```python
from build123d import *

# Parameters (mm, degrees)
F1_DEPTH       = 17
F3_W           = 0.5
F3_H           = 0.6
F4_DEPTH       = 5
F3_W_2         = 1
F3_H_2         = 1.2
F5_DEPTH       = 7
F7_W           = 2.5
F7_H           = 0.8
F8_DEPTH       = 37.3
F6_W           = 37.3
F6_H           = 12.9
F9_DEPTH       = 0.8
F10_W          = 9.4
F10_H          = 0.8
F11_DEPTH      = 36.4
F12_DEPTH      = 25
F12_DEPTH_BACK = 36.401
F13_DEPTH      = 0.901
F14_R          = 2


with BuildPart() as f1:
    # F0 (on Top) → F1 (new body)
    with BuildSketch(Plane.XY):
        Polygon((-0.9, 0), (0, 0), (0, 14), (35.5, 14), (35.5, 0), (36.4, 0), (36.4, 14.9), (-0.9, 14.9), align=None)
    extrude(amount=F1_DEPTH)

    # F3 (on offset) → F4 (join)
    with BuildSketch(Plane.XZ.offset(-1)):
        with Locations((0.25, 14.7)):
            Rectangle(F3_W, F3_H)
        with Locations((0.25, 7.05)):
            Rectangle(F3_W, F3_H)
    extrude(amount=-F4_DEPTH)

    # F3 (on offset) → F5 (cut)
    with BuildSketch(Plane.XZ.offset(-1)):
        with Locations((36, 14.8)):
            Rectangle(F3_W_2, F3_H_2)
        with Locations((36, 6.8)):
            Rectangle(F3_W_2, F3_H_2)
    extrude(amount=-F5_DEPTH, mode=Mode.SUBTRACT)

    # F7 (on face) → F8 (join, through all)
    with BuildSketch(Plane.YZ.offset(36.4)):
        with Locations((13.65, 4.6)):
            Rectangle(F7_W, F7_H)
    extrude(amount=-F8_DEPTH)

    # F6 (on face) → F9 (join)
    with BuildSketch(Plane.XY.offset(17)):
        with Locations((17.75, 8.45)):
            Rectangle(F6_W, F6_H)
    extrude(amount=F9_DEPTH)

    # F10 (on face) → F11 (join, through all)
    with BuildSketch(Plane(origin=(35.5, 0, 0), x_dir=(0, -1, 0), z_dir=(-1, 0, 0))):
        with Locations((-4.7, 1.6)):
            Rectangle(F10_W, F10_H)
        Polygon((-12.4, 4.2), (-9.4, 1.2), (-9.4, 2), (-12.4, 5), align=None)
    extrude(amount=F11_DEPTH)

    # F12 (cut, two sides): a face of the model
    f12_faces = [f1.faces().sort_by_distance(p)[0] for p in [
        (35.5, 7, 0.1461642911),
    ]]
    extrude(f12_faces, amount=-F12_DEPTH, mode=Mode.SUBTRACT)
    extrude(f12_faces, amount=F12_DEPTH_BACK, mode=Mode.SUBTRACT)

    # F13 (cut, through all): a face of the model
    f13_faces = [f1.faces().sort_by_distance(p)[0] for p in [
        (17.75, 14, 2.1),
    ]]
    extrude(f13_faces, amount=-F13_DEPTH, mode=Mode.SUBTRACT)

    # F14
    f14_edges = [f1.edges().sort_by_distance(p)[0] for p in [
        (17.75, 14.9, 4.2),
        (17.75, 9.4, 1.2),
        (-0.9, 4.7, 1.2),
        (36.4, 4.7, 1.2),
        (-0.9, 10.9, 2.7),
        (36.4, 10.9, 2.7),
        (36.4, 14.9, 11),
        (-0.9, 14.9, 11),
        (36.4, 13.65, 4.2),
        (-0.9, 13.65, 4.2),
    ]]
    fillet(f14_edges, radius=F14_R)


solid = f1.part
```
For this review, take the finished solid that the model builds, in its own axes (mm). A direction names the side the tool comes from. Round coordinates to 2 decimals unless told otherwise and drop trailing zeros. Loops run counter-clockwise (first coordinate to the right, second up) from the corner with the lowest first, then second, coordinate; pieces in that order, holes last.
Q1. Mouldability with a two-part tool opening along Z and no side actions: class faces 1 (the face through (17.98, 9.33, 1.35)), 2 (the face through (36, 4, 6.2)), 3 (the face through (17, 9, 17.8)), 4 (the face through (18, 8, 17)) as +Z half, -Z half, draft (parallel to the pull), parting line (faces both ways), or undercut.
Result sheet:
face 1: -Z half
face 2: undercut
face 3: +Z half
face 4: undercut
Q2. Add section C-C on x = 24.5. Write out the cut boundary in (y, z).
Result sheet:
outline: (0, 1.2) - (8.57, 1.2) arc R2 ccw to (9.99, 1.79) - (12.4, 4.2) - (12.9, 4.2) arc R2 ccw to (14.9, 6.2) - (14.9, 17.8) - (2, 17.8) - (2, 17) - (14, 17) - (14, 5) - (12.4, 5) - (9.4, 2) - (0, 2) - close
Q3. Insertion check: pin 1 Ø0.7 at (x, y) = (0, 0.5) entering from +Z; pin 2 Ø1 at (x, z) = (36, 15) entering from +Y; pin 3 Ø5 at (x, z) = (20, 10.5) entering from -Y. Each pin has a flat end and moves straight along its axis. Give the tip position at first contact, or say it passes through.
Result sheet:
pin 1: stops at z = 17
pin 2: stops at y = 14.57
pin 3: stops at y = 14
Q4. Machinability: for faces 5 (the face through (36, 12.4, 5)), 6 (the face through (18, 10.9, 3.5)), 7 (the face through (36, 8, 7)), 8 (the face through (36, 1, 17)), which of the approach directions +Z, -Z, +X, -X, +Y, -Y give a long, thin tool a straight path to every point of the face, cutting with its end or side? Answer none if there is none.
Result sheet:
face 5: -Z, +X, +Y
face 6: -Y
face 7: +X
face 8: +Z, +X, -X, -Y
Q5. To check wall thickness, follow line 1 along X through (y, z) = (6.5, 3.75); line 2 along Z through (x, y) = (29.5, 7.5); line 3 along Y through (x, z) = (24, 7). State the ranges of each line that lie inside material, in increasing order.
Result sheet:
line 1: x = -0.9 to 0, 35.5 to 36.4
line 2: z = 1.2 to 2, 17 to 17.8
line 3: y = 14 to 14.9
Q6. Add section B-B on z = 9. Write out the cut boundary in (x, y), plus the area to 3 significant figures.
Result sheet:
outline: (-0.9, 0) - (0, 0) - (0, 14) - (35.5, 14) - (35.5, 0) - (36.4, 0) - (36.4, 12.9) arc R2 ccw to (34.4, 14.9) - (1.1, 14.9) arc R2 ccw to (-0.9, 12.9) - close
area: 57.1 mm2
Q7. Add section A-A on y = 5. Write out the cut boundary in (x, z), plus the area to 3 significant figures.
Result sheet:
outline: (-0.9, 3.2) arc R2 ccw to (1.1, 1.2) - (34.4, 1.2) arc R2 ccw to (36.4, 3.2) - (36.4, 6.2) - (35.5, 6.2) - (35.5, 2) - (0, 2) - (0, 6.75) - (0.5, 6.75) - (0.5, 7.35) - (0, 7.35) - (0, 14.4) - (0.5, 14.4) - (0.5, 15) - (0, 15) - (0, 17) - (35.5, 17) - (35.5, 15.4) - (36.4, 15.4) - (36.4, 17.8) - (-0.9, 17.8) - close; (35.5, 7.4) - (36.4, 7.4) - (36.4, 14.2) - (35.5, 14.2) - close
area: 83.4 mm2
Q8. Add section D-D on y = 13.5. Write out the cut boundary in (x, z).
Result sheet:
outline: (-0.81, 6.2) arc R1.91 ccw to (1.1, 4.29) - (34.4, 4.29) arc R1.91 ccw to (36.31, 6.2) - (36.31, 17.8) - (-0.81, 17.8) - close; hole (0, 5) - (35.5, 5) - (35.5, 17) - (0, 17) - close
